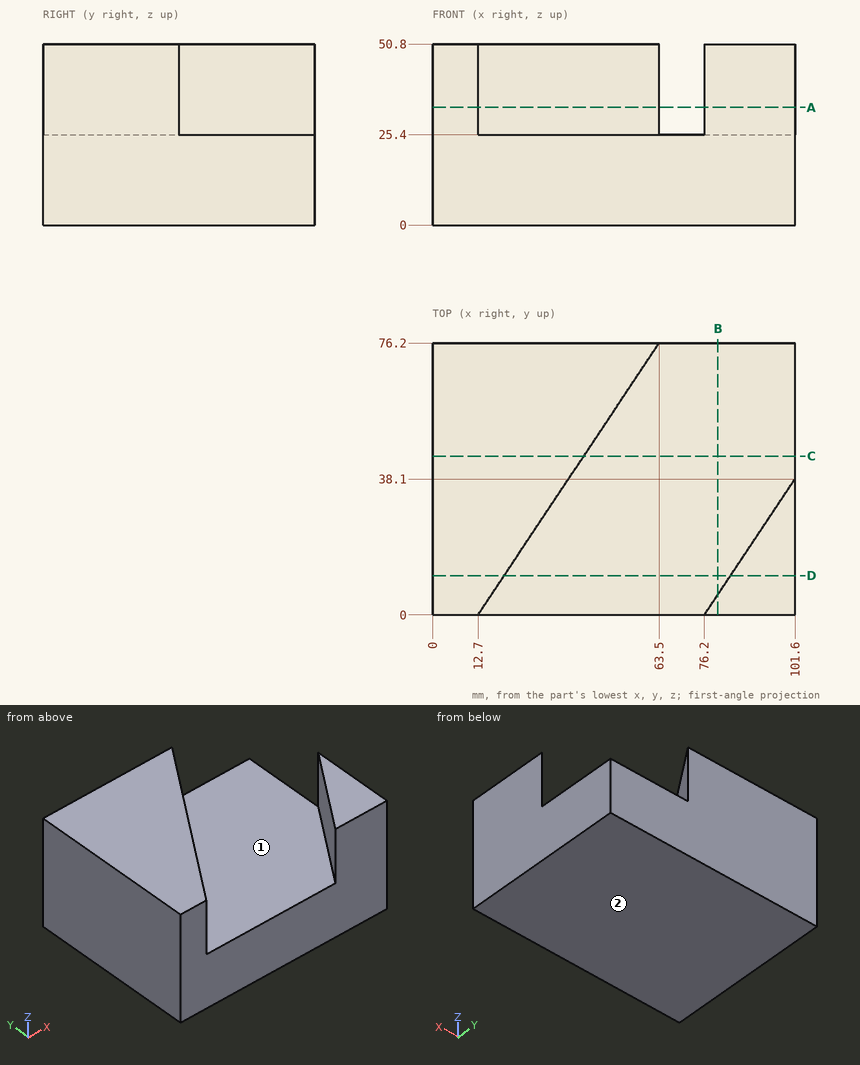
Can you work these out from the drawing? Everything is in mm from the part's minimum corner. A direction names the side the tool comes from. Coordinates: 2 decimals unless noted, no trailing zeros. Order: outer loops, then holes, each group sorted by start corner. A loop starts at its lowest first (then second) coordinate and runs counter-clockwise, first axis right, second up. Notation, with made-up numbers: (50.25, -6) -> (62.25, -6) arc R13 cw to (62.25, 4) -> close; hole circle Ø10 at (12, -19.75). An arc over 180 degrees is marked (long way). Use one line per item in the form item = value.
Q1. I need wall thicknesses on L1, parallel to Z at x = 53, y = 13; L2, parallel to X at y = 20, z = 34.5; L3, parallel to X at y = 50, z = 37.5. Which ranges of each line are inside material? Lowest first, please.
From the geometry:
L1 = 0 to 25.4
L2 = 0 to 26.03, 89.53 to 101.6
L3 = 0 to 46.03
Q2. Imagine slicing it at D-D, the plane y = 11. List the corners of the cut face in (x, z) for me.
From the geometry:
outline = (0, 0) -> (101.6, 0) -> (101.6, 50.8) -> (83.53, 50.8) -> (83.53, 25.4) -> (20.03, 25.4) -> (20.03, 50.8) -> (0, 50.8) -> close
Q3. Imagine slicing it at C-C, the plane y = 44.5. List the corners of the cut face in (x, z) for me, then the cut area to 3 significant figures.
From the geometry:
outline = (0, 0) -> (101.6, 0) -> (101.6, 25.4) -> (42.37, 25.4) -> (42.37, 50.8) -> (0, 50.8) -> close
area = 3,660 mm²
Q4. Imagine slicing it at B-B, the plane x = 80. List the corners of the cut face in (y, z) for me, then the cut area to 3 significant figures.
From the geometry:
outline = (0, 0) -> (76.2, 0) -> (76.2, 25.4) -> (5.7, 25.4) -> (5.7, 50.8) -> (0, 50.8) -> close
area = 2,080 mm²
Q5. Imagine slicing it at A-A, the plane z = 33. List the corners of the cut face in (x, y) for me.
From the geometry:
outline = (0, 0) -> (12.7, 0) -> (63.5, 76.2) -> (0, 76.2) -> close; (76.2, 0) -> (101.6, 0) -> (101.6, 38.1) -> close
Q6. Which directions (+Z, -Z, +X, -X, +Y, -Y) give clear straight access to the entire face, cutting with the end or side of a thin tool? Please do the marked faces 1 and 2.
From the geometry:
face_1 = +Z
face_2 = -Z, +X, -X, +Y, -Y
Q7. Will these pins go through, and if not, where does the flat tip stop? P1, Ø8, axis at x = 18.5, z = 34, coming from the -Y side; P2, Ø6, axis at x = 28, z = 28.5, coming from the -Y side; P3, Ø6, axis at x = 53, y = 49, coming from the +Z side.
From the geometry:
P1 = 2.7
P2 = 18.45
P3 = 25.4
